Source: three-view drawing plus pictorial views. Frame: mm from the lowest corner of the part. A direction names the side the tool comes from. Give positions to 0.01 mm unless a question says otherwise; leave off trailing zeros. Loops run counter-clockwise (first coordinate to the right, second up) from the corner with the lowest first, then second, coordinate; pieces in that order, holes last. Notation, with made-up numbers: M -2.75,42 L 33.25,42 A20 cw 33.25,52 Z; hole C 34,70 d9. An arc over 180 degrees is marked long. Answer as a JSON object with one key per item and string values. Group by question number.
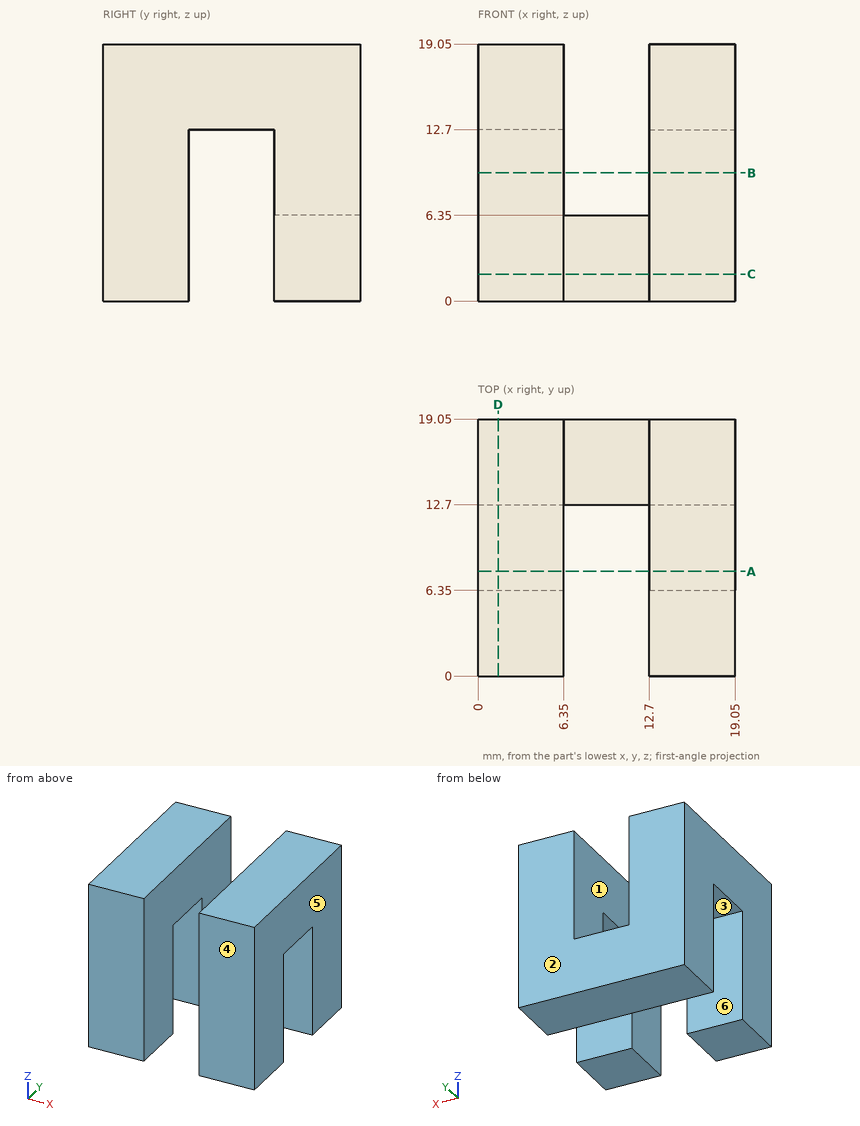
1. Section C-C (z = 2). Output: boundary loops of the cut face in (x, y), then the cut area to 3 significant figures.
2. Reachability of the marked faces 1, 2 and 3 from +Z, -Z, +X, -X, +Y, -Y: full face, straight path, thin tool, end or side. Return the list, or none.
3. Section B-B (z = 9.5). Output: boundary loops of the cut face in (x, y), then the cut area to 3 significant figures.
4. First-contact query: P1, Ø5, axis at x = 2.5, y = 9.5, coming from the -Z side; P2, Ø3, axis at x = 9.5, y = 16, coming from the +Z side. Flat tips, straight axial feed; report the tip coordinate or a pass-through.
5. Material intervals for L1, parallel to X at y = 15.75, z = 12.5; L2, parallel to Z at x = 1.25, y = 8.5, sorted ascending.
6. Section A-A (y = 7.75). Output: boundary loops of the cut face in (x, z).
7. Mould query, pull axis Y, two halves, no side actions, for the marked faces 4, 5 and 6. Classes: pulls with the +Y half, pulls with the -Y half, needs draft (parallel to the pull), parting line crosses it, or undercut.
8. Section D-D (x = 1.5). Output: boundary loops of the cut face in (y, z), then the cut area to 3 significant figures.
Geometry results:
{
 "1": {"outline": "M 0,0 L 6.35,0 L 6.35,6.35 L 0,6.35 Z; M 0,12.7 L 19.05,12.7 L 19.05,19.05 L 0,19.05 Z; M 12.7,0 L 19.05,0 L 19.05,6.35 L 12.7,6.35 Z", "area": "202 mm2"},
 "2": {"face 1": "+Z, -Y", "face 2": "+Z, -Z, +X, -X, +Y", "face 3": "-Z, +X, -X"},
 "3": {"outline": "M 0,0 L 6.35,0 L 6.35,6.35 L 0,6.35 Z; M 0,12.7 L 6.35,12.7 L 6.35,19.05 L 0,19.05 Z; M 12.7,0 L 19.05,0 L 19.05,6.35 L 12.7,6.35 Z; M 12.7,12.7 L 19.05,12.7 L 19.05,19.05 L 12.7,19.05 Z", "area": "161 mm2"},
 "4": {"P1": "z = 12.7", "P2": "z = 6.35"},
 "5": {"L1": "0 to 6.35, 12.7 to 19.05", "L2": "12.7 to 19.05"},
 "6": {"outline": "M 0,12.7 L 6.35,12.7 L 6.35,19.05 L 0,19.05 Z; M 12.7,12.7 L 19.05,12.7 L 19.05,19.05 L 12.7,19.05 Z"},
 "7": {"face 4": "pulls with the -Y half", "face 5": "needs draft", "face 6": "undercut"},
 "8": {"outline": "M 0,0 L 6.35,0 L 6.35,12.7 L 12.7,12.7 L 12.7,0 L 19.05,0 L 19.05,19.05 L 0,19.05 Z", "area": "282 mm2"}
}
